```python
from build123d import *

# Parameters (mm, degrees)
F2_R     = 2.25
F3_DEPTH = 25
F2_R_2   = 4.25
F4_DEPTH = 2
F5_SIZE  = 1


with BuildPart() as f1:
    # F0 (on Front) → F1 (revolve)
    with BuildSketch(Plane.XZ):
        with BuildLine():
            Line((65, -5.5), (65, 0))
            Line((65, 0), (29.289105, 0))
            add(Edge.make_bspline(
                [(21.75, -6.322154), (22.552238, -4.150534), (26.594359, 0), (29.289105, 0)],
                knots=[0, 0, 0, 0, 9.839092, 9.839092, 9.839092, 9.839092], degree=3))
            Line((21.75, -6.322154), (18.75, -6.322154))
            add(Edge.make_bspline(
                [(0, 12.427846), (11.965546, 12.285027), (18.75, 0), (18.75, -6.322154)],
                knots=[0, 0, 0, 0, 26.516504, 26.516504, 26.516504, 26.516504], degree=3))
            Line((0, 12.427846), (0, -13.315069))
            Line((0, -13.315069), (45, -13.315069))
            Line((45, -13.315069), (45, -5.5))
            Line((45, -5.5), (65, -5.5))
        make_face()
    revolve(axis=Axis((0, 0, -0.443612), (0, 0, 1)))

    # F2 (on face) → F3 (cut)
    with BuildSketch(Plane.XY):
        with Locations((-50.44598, 29.125)):
            Circle(F2_R)
        with Locations((0, 58.25)):
            Circle(F2_R)
        with Locations((50.44598, 29.125)):
            Circle(F2_R)
        with Locations((50.44598, -29.125)):
            Circle(F2_R)
        with Locations((0, -58.25)):
            Circle(F2_R)
        with Locations((-50.44598, -29.125)):
            Circle(F2_R)
    extrude(amount=-F3_DEPTH, mode=Mode.SUBTRACT)

    # F2 (on face) → F4 (cut)
    with BuildSketch(Plane.XY):
        with Locations((-50.44598, 29.125)):
            Circle(F2_R_2)
        with Locations((-50.44598, 29.125)):
            Circle(F2_R, mode=Mode.SUBTRACT)
        with Locations((0, 58.25)):
            Circle(F2_R_2)
        with Locations((0, 58.25)):
            Circle(F2_R, mode=Mode.SUBTRACT)
        with Locations((50.44598, 29.125)):
            Circle(F2_R_2)
        with Locations((50.44598, 29.125)):
            Circle(F2_R, mode=Mode.SUBTRACT)
        with Locations((50.44598, -29.125)):
            Circle(F2_R_2)
        with Locations((50.44598, -29.125)):
            Circle(F2_R, mode=Mode.SUBTRACT)
        with Locations((0, -58.25)):
            Circle(F2_R_2)
        with Locations((0, -58.25)):
            Circle(F2_R, mode=Mode.SUBTRACT)
        with Locations((-50.44598, -29.125)):
            Circle(F2_R_2)
        with Locations((-50.44598, -29.125)):
            Circle(F2_R, mode=Mode.SUBTRACT)
    extrude(amount=-F4_DEPTH, mode=Mode.SUBTRACT)

    # F5
    f5_edges = [f1.edges().sort_by_distance(p)[0] for p in [
        (-65, 0, 0),
    ]]
    chamfer(f5_edges, length=F5_SIZE)


solid = f1.part
```
The listing builds one solid part. Answer for the finished solid, in the listing's coordinates (mm). A direction names the side the tool comes from. Coordinates: 2 decimals unless noted, no trailing zeros. Answer as a JSON object with one key per item and string values. Group by question number.
1. Flat-ended cylindrical pins translate along their axes: P1, Ø2.5, axis at x = 50.45, y = 29.12, coming from the +Z side; P2, Ø2.5, axis at x = 1.5, y = 57, coming from the +Z side; P3, Ø9.5, axis at x = -1, y = -58.5, coming from the +Z side; P4, Ø10, axis at y = -49, z = -5.5, coming from the -X side. Find the tip coordinate at first contact, or state that the pin passes through.
2. A tool of negligible diameter and unlimited length cuts with its end or side. For faces 4 (the cylindrical face through (-1.8, -59.6, -3.7)), 5 (the cylindrical face through (-0.92, 54.1, -0.99)), from which of +Z, -Z, +X, -X, +Y, -Y can it reach the whole face along a straight path? Write none if from no direction.
3. Straight lines are drawn through the part: line 1 (Y direction, x = 0, z = -0.6); line 2 (Z direction, x = 10, y = 30.5); line 3 (Y direction, x = 0, z = -0.55). For each, find the intervals that lie inside material, in ascending order.
4. Determine the mould class of faces 1 (the flat face through (6, 18, -6.322)), 2 (the flat face through (1, 1, -13.315)), 3 (the cylindrical face through (20.765, -39.923, -9.353)) for opening direction X: released by +X, released by -X, zero draft, split by the parting line, or undercut.
Values follow:
{
 "1": {"P1": "through", "P2": "z = -2", "P3": "z = 0", "P4": "x = -47.84"},
 "2": {"face 4": "+Z, -Z", "face 5": "+Z"},
 "3": {"line 1": "-64.6 to -62.5, -54 to -27.24, -17.44 to 17.44, 27.24 to 54, 62.5 to 64.6", "line 2": "-13.32 to 0", "line 3": "-64.55 to -62.5, -54 to -27.34, -17.42 to 17.42, 27.34 to 54, 62.5 to 64.55"},
 "4": {"face 1": "undercut", "face 2": "zero draft", "face 3": "split by the parting line"}
}
